from build123d import *

# Parameters (mm, degrees)
F1_DEPTH = 2.286
F2_T     = -2.54
F4_D     = 1.016
F4_DEPTH = 18.034
F4_TIP   = 0.3052371945


with BuildPart() as f1:
    # F0 (on Right) → F1 (new body)
    with BuildSketch(Plane.YZ):
        with BuildLine():
            Line((-35.6506742537, 8.3372171661), (-74.139625051, 8.3372171661))
            Line((-74.139625051, 8.3372171661), (-74.139625051, -5.7919719098))
            Line((-74.139625051, -5.7919719098), (-44.5406742537, -5.7919719098))
            ThreePointArc((-44.5406742537, -5.7919719098), (-38.254494969, -3.1881511945), (-35.6506742537, 3.0980280902))
            Line((-35.6506742537, 3.0980280902), (-35.6506742537, 8.3372171661))
        make_face()
        Polygon((-27.7069620788, 8.3372171661), (-35.6506742537, 3.0980280902), (-27.7069620788, 3.0980280902), align=None)
        Polygon((-27.7069620788, 8.3372171661), (-35.6506742537, 8.3372171661), (-35.6506742537, 3.0980280902), align=None)
    extrude(amount=F1_DEPTH)

    # F2
    f2_openings = [f1.faces().sort_by_distance(p)[0] for p in [
        (2.286, -53.710375, 1.749572),
        (0, -53.710375, 1.749572),
    ]]
    offset(amount=F2_T, openings=f2_openings, kind=Kind.INTERSECTION)

    # F4
    with Locations(Plane(origin=(0, -27.7069620788, 0), x_dir=(-1, 0, 0), z_dir=(0, 1, 0))):
        with Locations((-1.1559764389, 7.2045344859), (-1.1559764389, 5.5570374243), (-1.1559764389, 4.1465191171)):
            Hole(F4_D / 2, depth=F4_DEPTH)
            with Locations((0, 0, -(F4_DEPTH + F4_TIP / 2))):  # 118° drill point
                Cone(0, F4_D / 2, F4_TIP, mode=Mode.SUBTRACT)


solid = f1.part
The model under review builds one solid part; all positions refer to its coordinate system, in mm. A direction names the side the tool comes from. Round coordinates to 2 decimals unless told otherwise and drop trailing zeros. Order: outer loops, then holes, each group sorted by start corner. A loop starts at its lowest first (then second) coordinate and runs counter-clockwise, first axis right, second up. Notation, with made-up numbers: (-9.75, 47.25) - (2.25, 47.25) arc R25 ccw to (2.25, 61.25) - close; hole circle Ø2 at (35, -15). An arc over 180 degrees is marked (long way). Use one line per item in the form item = value.
Q1. Add section B-B on y = -60. Give the boundary of the cut face in (x, z).
Response values:
outline = (0, -5.79) - (2.29, -5.79) - (2.29, -3.25) - (0, -3.25) - close; (0, 5.8) - (2.29, 5.8) - (2.29, 8.34) - (0, 8.34) - close
Q2. Add section A-A on y = -43. Give the boundary of the cut face in (x, z).
Response values:
outline = (0, -5.66) - (2.29, -5.66) - (2.29, -3.06) - (0, -3.06) - close; (0, 5.8) - (0.71, 5.8) arc R0.51 cw to (1.6, 5.8) - (2.29, 5.8) - (2.29, 8.34) - (0, 8.34) - close; hole circle Ø1.02 at (1.16, 7.2)
Q3. Add section C-C on z = 1.25. Give the boundary of the cut face in (x, y), then the cut area to 3 significant figures.
Response values:
outline = (0, -74.14) - (2.29, -74.14) - (2.29, -71.6) - (0, -71.6) - close; (0, -38.47) - (2.29, -38.47) - (2.29, -35.84) - (0, -35.84) - close
area = 11.8 mm^2
Q4. To check wall thickness, follow line 1 (Z direction, x = 1.25, y = -42.5); line 2 (Z direction, x = 1.1, y = -64); line 3 (Z direction, x = 1.3, y = -41). State the ranges of each line that lie inside material, in increasing order.
Response values:
line_1 = -5.55 to -2.92, 6.06 to 6.71, 7.7 to 8.34
line_2 = -5.79 to -3.25, 5.8 to 8.34
line_3 = -5.06 to -2.17, 6.04 to 6.72, 7.69 to 8.34
Q5. Mouldability with a two-part tool opening along Y and no side actions: class faces 4 (the flat face through (1, -71.6, 1)), 5 (the cylindrical face through (1.127, -39.277, -0.453)), 6 (the cylindrical face through (1.09, -36.85, 7.71)), 7 (the conical face through (1.115, -45.993, 7.126)) as pulls with the +Y half, pulls with the -Y half, needs draft (parallel to the pull), parting line crosses it, or undercut.
Response values:
face_4 = undercut
face_5 = undercut
face_6 = needs draft
face_7 = pulls with the +Y half
Q6. Tool access review of faces 1 (the flat face through (1, -32, 3.098)), 2 (the cylindrical face through (1.09, -33.12, 4.65)), 3 (the flat face through (1, -58, -3.252)): name each direction out of +Z, -Z, +X, -X, +Y, -Y from which nothing blocks a thin tool from reaching the whole face with its end or side.
Response values:
face_1 = -Z, +X, -X, +Y
face_2 = +Y
face_3 = +X, -X
Q7. Clearance check with flat-ended pins moving along their axes: P1, Ø0.6, axis at x = 1.16, z = 4.15, coming from the +Y side; P2, Ø0.7, axis at x = 1, z = -0.5, coming from the +Y side. State where each tip first meets the part, or that it passes through.
Response values:
P1 = -71.6
P2 = -36.27
